from build123d import *

# Parameters (mm, degrees)
SKETCH_1_W          = 60
SKETCH_1_H          = 35
EXTRUDE_1_DEPTH     = 20
HOLE_WIZARD_356_D   = 9
HOLE_WIZARD_461_D   = 8.2
SKETCH_8_W          = 2.7
SKETCH_8_H          = 5.7
CUT_EXTRUDE_1_DEPTH = 41.078048855
SKETCH_9_R          = 1.6
CUT_EXTRUDE_2_DEPTH = 10
SKETCH_10_W         = 60
SKETCH_10_H         = 20
EXTRUDE_2_DEPTH     = 14.25


with BuildPart() as part:
    # 草图1 → 凸台-拉伸1 (new body)
    with BuildSketch(Plane.XY):
        Rectangle(SKETCH_1_W, SKETCH_1_H)
    extrude(amount=EXTRUDE_1_DEPTH)

    # Hole Wizard 356 (through all)
    with Locations(Plane.XY.offset(20)):
        with Locations((0, 0)):
            Hole(HOLE_WIZARD_356_D / 2)

    # Hole Wizard 461 (through all)
    with Locations(Plane.XY.offset(20)):
        with Locations((20, 0), (-20, 0)):
            Hole(HOLE_WIZARD_461_D / 2)

    # 草图8 → 切除-拉伸1 (cut, through all)
    with BuildSketch(Plane.XY.offset(20)):
        with Locations((27.05, 0)):
            Rectangle(SKETCH_8_W, SKETCH_8_H)
    cut_extrude_1 = extrude(amount=-CUT_EXTRUDE_1_DEPTH, mode=Mode.SUBTRACT)

    # 草图9 → 切除-拉伸2 (cut)
    with BuildSketch(Plane(origin=(30, 0, 0), x_dir=(0, 0, -1), z_dir=(1, 0, 0))):
        with Locations(Location((-10, 0, 0), (0, 0, 180))):
            Circle(SKETCH_9_R)
    cut_extrude_2 = extrude(amount=-CUT_EXTRUDE_2_DEPTH, mode=Mode.SUBTRACT)

    # 镜向1: 切除-拉伸1, 切除-拉伸2 across plane
    add(cut_extrude_1.mirror(Plane(origin=(0, 0, 0), x_dir=(0, 0, 1), z_dir=(1, 0, 0))), mode=Mode.SUBTRACT)
    add(cut_extrude_2.mirror(Plane(origin=(0, 0, 0), x_dir=(0, 0, 1), z_dir=(1, 0, 0))), mode=Mode.SUBTRACT)

    # 草图10 → 凸台-拉伸2 (add)
    with BuildSketch(Plane(origin=(0, 17.5, 0), x_dir=(1, 0, 0), z_dir=(0, 1, 0))):
        with Locations((0, -10)):
            Rectangle(SKETCH_10_W, SKETCH_10_H)
    extrude(amount=EXTRUDE_2_DEPTH)


solid = part.part
Check sheet for the modelled part. Datum: model origin and axes. Units: mm. A direction names the side the tool comes from. Coordinates: 2 decimals unless noted, no trailing zeros. Write each loop counter-clockwise with the first axis right and the second up, starting at its lowest first coordinate (ties: lowest second). Pieces come first, ordered by that corner, then holes.
Item 1: Access from +Z, -Z, +X, -X, +Y, -Y to the whole of each face (thin tool, end or side, straight path). Record for faces 4 (the face through (27, -2.85, 10)), 5 (the face through (29.21, -0.07, 8.4)), 6 (the face through (0, 31.75, 10)), 7 (the face through (0, 7, 0)), 8 (the face through (-29.21, -0.07, 8.4)).
Numbers:
face 4: +Z, -Z
face 5: +X
face 6: +Z, -Z, +X, -X, +Y
face 7: -Z, +X, -X, +Y, -Y
face 8: -X
Item 2: Cross-section at A-A on x = -20. Record the boundary of the cut face in (y, z).
Numbers:
outline: (-17.5, 0) - (-4.1, 0) - (-4.1, 20) - (-17.5, 20) - close; (4.1, 0) - (31.75, 0) - (31.75, 20) - (4.1, 20) - close
Item 3: Depth check by flat-ended pin: pin 1 Ø3 at (y, z) = (0, 10) entering from +X; pin 2 Ø1.9 at (y, z) = (0, 10) entering from +X; pin 3 Ø1.9 at (y, z) = (0, 10) entering from -X. Enter the tip coordinate at first touch or a pass-through.
Numbers:
pin 1: stops at x = 16.18
pin 2: stops at x = 16.01
pin 3: stops at x = -16.01
Item 4: Cross-section at D-D on x = 0. Record the boundary of the cut face in (y, z).
Numbers:
outline: (-17.5, 0) - (-4.5, 0) - (-4.5, 20) - (-17.5, 20) - close; (4.5, 0) - (31.75, 0) - (31.75, 20) - (4.5, 20) - close
Item 5: Mould release check, pull along Z, two halves, no side actions. Record for faces 1 (the face through (24.751, -0.481, 11.526)), 2 (the face through (-27, 2.85, 10)), 3 (the face through (0, 7, 20)): released by +Z, released by -Z, zero draft, split by the parting line, or undercut.
Numbers:
face 1: undercut
face 2: zero draft
face 3: released by +Z
Item 6: Cross-section at C-C on z = 6. Record the boundary of the cut face in (x, y).
Numbers:
outline: (-30, -17.5) - (30, -17.5) - (30, 31.75) - (-30, 31.75) - close; hole (-28.4, -2.85) - (-25.7, -2.85) - (-25.7, 2.85) - (-28.4, 2.85) - close; hole circle Ø8.2 at (-20, 0); hole circle Ø9 at (0, 0); hole circle Ø8.2 at (20, 0); hole (25.7, -2.85) - (28.4, -2.85) - (28.4, 2.85) - (25.7, 2.85) - close
Item 7: Scan lines: probe 1 along Y at (x, z) = (29.5, 10); probe 2 along Y at (x, z) = (0, 15.5); probe 3 along X at (y, z) = (3.5, 13). Record each from-to range of solid material in increasing order.
Numbers:
probe 1: y = -17.5 to -1.6, 1.6 to 31.75
probe 2: y = -17.5 to -4.5, 4.5 to 31.75
probe 3: x = -30 to -22.14, -17.86 to -2.83, 2.83 to 17.86, 22.14 to 30
